```python
from build123d import *

# Parameters (mm, degrees)
F0_W      = 227.177798748
F0_H      = 67.4825310707
F0_W_2    = 7.6686143875
F0_W_3    = 40.7849550247
F0_H_2    = 19.1998630762
F1_DEPTH  = 25.4
F2_W      = 713.7889862061
F2_H      = 722.4479019642
F3_DEPTH  = 10751.3055801392
F5_W      = 833.6800336838
F5_H      = 828.9024829865
F6_DEPTH  = 25.4
F7_W      = 833.6800336838
F7_H      = 828.9024829865
F7_R      = 213.8106585198
F8_DEPTH  = 25.4
F9_W      = 805.6761920452
F9_H      = 828.9024829865
F9_R      = 212.5191058953
F9_W_2    = 28.0038416386
F10_DEPTH = 25.4
F11_W     = 833.6800336838
F11_H     = 828.9024829865
F11_R     = 151.5456161356
F12_DEPTH = 25.4
F13_W     = 680.4287135601
F13_H     = 667.77536273
F13_R     = 210.9258695705
F14_DEPTH = 25.4
F15_W     = 153.2513201237
F15_H     = 667.77536273
F16_DEPTH = 25.4
F17_W     = 371.1061030626
F17_H     = 256.3967704773
F17_W_2   = 32.0261418819
F17_H_2   = 25.0417590141
F17_W_3   = 119.3500384688
F17_H_3   = 111.177533865
F18_DEPTH = 25.4


with BuildPart() as f1:
    # F0 (on Right) → F1 (new body)
    with BuildSketch(Plane.YZ):
        Polygon((-598.1872081757, 183.7075799704), (-598.1872081757, 196.1238980293), (-605.8558225632, 196.1238980293), (-605.8558225632, 145.6781327724), (-598.1872081757, 145.6781327724), align=None)
        Polygon((-605.8558225632, 196.1238980293), (-598.1872081757, 196.1238980293), (-598.1872081757, 401.8925428391), (-605.8558225632, 401.8925428391), (-605.8558225632, 215.3237611055), align=None)
        Polygon((-1197.3617076874, 196.1238980293), (-605.8558225632, 196.1238980293), (-605.8558225632, 215.3237611055), (-1548.1258630753, 215.3237611055), (-1548.1258630753, 196.1238980293), align=None)
        Polygon((698.481798172, 183.7075799704), (-598.1872081757, 183.7075799704), (-598.1872081757, 145.6781327724), (-598.1872081757, 78.1956017017), (-598.1872081757, 8.7382793427), (698.481798172, 8.7382793427), align=None)
        Polygon((-1197.3617076874, 145.6781327724), (-1197.3617076874, 196.1238980293), (-1548.1258630753, 196.1238980293), (-1548.1258630753, 78.1956017017), (-833.0336213112, 78.1956017017), (-833.0336213112, 145.6781327724), align=None)
        with Locations((-719.4447219372, 111.9368672371)):
            Rectangle(F0_W, F0_H)
        with Locations((-602.0215153694, 111.9368672371)):
            Rectangle(F0_W_2, F0_H)
        Polygon((-1548.1258630753, 215.3237611055), (-605.8558225632, 215.3237611055), (-605.8558225632, 401.8925428391), (-1588.9108181, 401.8925428391), (-1588.9108181, 215.3237611055), align=None)
        with Locations((-1568.5183405876, 205.7238295674)):
            Rectangle(F0_W_3, F0_H_2)
    extrude(amount=F1_DEPTH)

    # F2 (on face) → F3 (join)
    with BuildSketch(Plane(origin=(0, 0, 0), x_dir=(0, -1, 0), z_dir=(-1, 0, 0))):
        with Locations((448.7802386284, 201.1957615614)):
            Rectangle(F2_W, F2_H)
    extrude(amount=F3_DEPTH)


with BuildPart() as f6:
    # F5 (on Right) → F6 (new body)
    with BuildSketch(Plane.YZ):
        with Locations((-1.6488134861, 0.6756186485)):
            Rectangle(F5_W, F5_H)
    extrude(amount=F6_DEPTH)

    # F7 (on face) → F8 (join)
    with BuildSketch(Plane.YZ.offset(25.4)):
        with Locations((-1.6488134861, 0.6756186485)):
            Rectangle(F7_W, F7_H)
        Circle(F7_R, mode=Mode.SUBTRACT)
    extrude(amount=F8_DEPTH)

    # F9 (on face) → F10 (join)
    with BuildSketch(Plane.YZ.offset(50.8)):
        with Locations((-15.6507343054, 0.6756186485)):
            Rectangle(F9_W, F9_H)
        Circle(F9_R, mode=Mode.SUBTRACT)
        with Locations((401.1892825365, 0.6756186485)):
            Rectangle(F9_W_2, F9_H)
    extrude(amount=F10_DEPTH)

    # F11 (on face) → F12 (join)
    with BuildSketch(Plane(origin=(0, 0, 0), x_dir=(0, -1, 0), z_dir=(-1, 0, 0))):
        with Locations((1.6488134861, 0.6756186485)):
            Rectangle(F11_W, F11_H)
        Circle(F11_R, mode=Mode.SUBTRACT)
    extrude(amount=F12_DEPTH)

    # F13 (on face) → F14 (join)
    with BuildSketch(Plane(origin=(-25.4, 0, 0), x_dir=(0, -1, 0), z_dir=(-1, 0, 0))):
        with Locations((-74.9768465757, -79.8879414797)):
            Rectangle(F13_W, F13_H)
        Circle(F13_R, mode=Mode.SUBTRACT)
    extrude(amount=F14_DEPTH)

    # F15 (on face) → F16 (join)
    with BuildSketch(Plane(origin=(-25.4, 0, 0), x_dir=(0, -1, 0), z_dir=(-1, 0, 0))):
        Polygon((418.488830328, 415.1268601418), (-415.1912033558, 415.1268601418), (-415.1912033558, 253.9997398853), (265.2375102043, 253.9997398853), (418.488830328, 253.9997398853), align=None)
        with Locations((341.8631702662, -79.8879414797)):
            Rectangle(F15_W, F15_H)
    extrude(amount=F16_DEPTH)

    # F17 (on face) → F18 (join)
    with BuildSketch(Plane(origin=(-50.8, 0, 0), x_dir=(0, -1, 0), z_dir=(-1, 0, 0))):
        with Locations((232.9357787967, 543.3252453804)):
            Rectangle(F17_W, F17_H)
        Polygon((418.488830328, 415.1268601418), (47.3827272654, 415.1268601418), (47.3827272654, 671.523630619), (-65.5413940549, 671.523630619), (-65.5413940549, 168.3508753777), (-65.5413940549, 57.1733415127), (-65.5413940549, -285.7585549355), (418.488830328, -285.7585549355), (418.488830328, -220.9893465042), (418.488830328, -194.4699287415), (418.488830328, 0.6756186485), align=None)
        with Locations((16.013070941, -182.512909174)):
            Rectangle(F17_W_2, F17_H_2, mode=Mode.SUBTRACT)
        Polygon((418.488830328, 671.523630619), (418.488830328, 415.1268601418), (421.7643141747, 415.1268601418), (421.7643141747, 1019.0404653549), (47.3827272654, 1019.0404653549), (47.3827272654, 671.523630619), align=None)
        Polygon((421.7643141747, 415.1268601418), (418.488830328, 415.1268601418), (418.488830328, 0.6756186485), (418.488830328, -194.4699287415), (748.2059001923, -194.4699287415), (748.2059001923, 415.1268601418), align=None)
        with Locations((-125.2164132893, 112.7621084452)):
            Rectangle(F17_W_3, F17_H_3)
    extrude(amount=F18_DEPTH)


solid = f6.part
```
Geometry: final body of the model. Coordinates: model frame, mm. A direction names the side the tool comes from. Coordinates: 2 decimals unless noted, no trailing zeros. Order: outer loops, then holes, each group sorted by start corner. A loop starts at its lowest first (then second) coordinate and runs counter-clockwise, first axis right, second up. Notation, with made-up numbers: M 61,13 L 86,13 A34 cw 86,43 Z; hole C 29,-39.5 d11. An arc over 180 degrees is marked long. Answer as CSV lines item,"result".
Q1. Draft query along Z for faces 4 (the flat face through (-50.8, -54, 3)), 5 (the flat face through (1, -418.489, -5)), 6 (the flat face through (14, -7, 415.127)). Return one class per face: pulls with the +Z half, pulls with the -Z half, needs draft (parallel to the pull), parting line crosses it, or undercut.
Answers:
face 4,"undercut"
face 5,"needs draft"
face 6,"pulls with the +Z half"
Q2. Section A-A on y = -334. Return the cut outline in (x, z), and give its area (3 significant figures).
Answers:
outline,"M -76.2,-285.76 L -50.8,-285.76 L -50.8,-413.78 L 76.2,-413.78 L 76.2,415.13 L -50.8,415.13 L -50.8,1019.04 L -76.2,1019.04 Z"
area,"138,000 mm^2"
Q3. Section D-D on y = -664. Return the cut outline in (x, z).
Answers:
outline,"M -76.2,-194.47 L -50.8,-194.47 L -50.8,415.13 L -76.2,415.13 Z"
Q4. First-contact query: P1, Ø12.5, axis at x = -68.5, y = -631.5, coming from the +Z side; P2, Ø20.5, axis at x = -64.5, y = -657, coming from the -Z side; P3, Ø10, axis at x = 10, z = 344, coming from the -Y side. Flat tips, straight axial feed; report the tip coordinate or a pass-through.
Answers:
P1,"stops at z = 415.13"
P2,"stops at z = -194.47"
P3,"stops at y = -418.49"
Q5. Set-up query: faces 1 (the flat face through (14, 415.191, 6)), 2 (the cylindrical face through (63.32, -27.67, 210.71)), 3 (the cylindrical face through (-12.522, -144.548, 45.52)). Return all of +Z, -Z, +X, -X, +Y, -Y with unobstructed straight access to the full face (end or side cutting, diameter ignored); none if empty.
Answers:
face 1,"+Z, -Z, +X, -X, +Y"
face 2,"+X"
face 3,"none"
Q6. Section C-C on z = -237. Return the cut outline in (x, y), and give its area (3 significant figures).
Answers:
outline,"M -76.2,-418.49 L 76.2,-418.49 L 76.2,415.19 L -50.8,415.19 L -50.8,65.54 L -76.2,65.54 Z"
area,"118,000 mm^2"
Q7. Line query: probe 1 along Z at (x, y) = (56, 0); probe 2 along Z at (x, y) = (-20, 0); probe 3 along Y at (x, z) = (53.5, 24.5). Output: solid intervals per line, ascending. Write a range as [from, to].
Answers:
probe 1,"z = [-413.78, -212.52], [212.52, 415.13]"
probe 2,"z = [-413.78, -151.55], [151.55, 415.13]"
probe 3,"y = [-418.49, -211.1], [211.1, 415.19]"
Q8. Section B-B on z = 0. Return the cut outline in (x, y), and give its area (3 significant figures).
Answers:
outline,"M -76.2,-748.21 L -50.8,-748.21 L -50.8,-418.49 L 76.2,-418.49 L 76.2,-212.52 L 50.8,-212.52 L 50.8,-213.81 L 25.4,-213.81 L 25.4,213.81 L 50.8,213.81 L 50.8,212.52 L 76.2,212.52 L 76.2,415.19 L -50.8,415.19 L -50.8,210.93 L -25.4,210.93 L -25.4,151.55 L 0,151.55 L 0,-151.55 L -25.4,-151.55 L -25.4,-210.93 L -50.8,-210.93 L -50.8,65.54 L -76.2,65.54 Z"
area,"86,500 mm^2"
